from build123d import *

# Parameters (mm, degrees)
SKETCH1_W            = 202.5
SKETCH1_H            = 75
BOSS_EXTRUDE7_DEPTH  = 2.5
SKETCH9_W            = 10
SKETCH9_H            = 2.5
BOSS_EXTRUDE8_DEPTH  = 2.5
SKETCH10_W           = 10
SKETCH10_H           = 2.5
BOSS_EXTRUDE9_DEPTH  = 2.5
SKETCH11_R           = 1.5
CUT_EXTRUDE3_DEPTH   = 2.5
SKETCH12_W           = 2.5
SKETCH12_H           = 55
BOSS_EXTRUDE10_DEPTH = 2.5
SKETCH13_W           = 2.5
SKETCH13_H           = 55
BOSS_EXTRUDE11_DEPTH = 3


with BuildPart() as part:
    # Sketch1 → Boss-Extrude7 (new body)
    with BuildSketch(Plane.XY):
        with Locations((101.25, 37.5)):
            Rectangle(SKETCH1_W, SKETCH1_H)
    extrude(amount=BOSS_EXTRUDE7_DEPTH)

    # Sketch9 → Boss-Extrude8 (add)
    with BuildSketch(Plane(origin=(0, 75, 0), x_dir=(1, 0, 0), z_dir=(0, 1, 0))):
        with Locations((197.5, -1.25)):
            Rectangle(SKETCH9_W, SKETCH9_H)
    extrude(amount=BOSS_EXTRUDE8_DEPTH)

    # Sketch10 → Boss-Extrude9 (add)
    with BuildSketch(Plane.XZ):
        with Locations((197.5, 1.25)):
            Rectangle(SKETCH10_W, SKETCH10_H)
    extrude(amount=BOSS_EXTRUDE9_DEPTH)

    # Sketch11 → Cut-Extrude3 (cut)
    with BuildSketch(Plane.XY.offset(2.5)):
        with Locations((188.75, 37.5)):
            Circle(SKETCH11_R)
    extrude(amount=-CUT_EXTRUDE3_DEPTH, mode=Mode.SUBTRACT)

    # Sketch12 → Boss-Extrude10 (add)
    with BuildSketch(Plane(origin=(0, 0, 0), x_dir=(-1, 0, 0), z_dir=(0, 0, -1))):
        with Locations((-1.25, 37.5)):
            Rectangle(SKETCH12_W, SKETCH12_H)
    extrude(amount=BOSS_EXTRUDE10_DEPTH)

    # Sketch13 → Boss-Extrude11 (add)
    with BuildSketch(Plane.ZY):
        with Locations((-1.25, 37.5)):
            Rectangle(SKETCH13_W, SKETCH13_H)
    extrude(amount=BOSS_EXTRUDE11_DEPTH)


solid = part.part
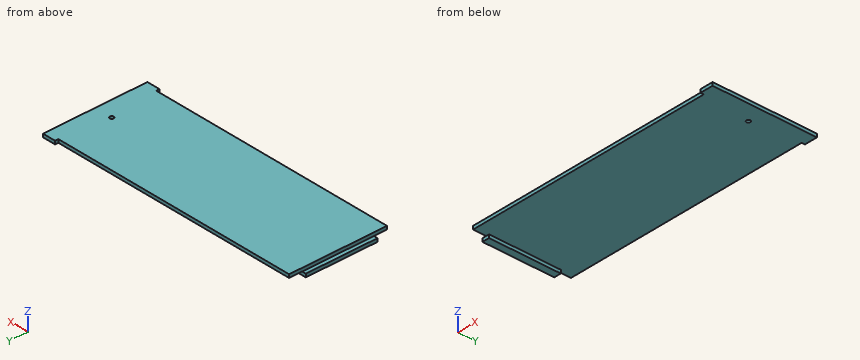
Source: CAD feature listing. Evaluate the final solid. Frame: model axes, mm. Give positions to 0.01 mm unless a question says otherwise; leave off trailing zeros. Write each loop counter-clockwise with the first axis right and the second up, starting at its lowest first coordinate (ties: lowest second). Pieces come first, ordered by that corner, then holes. Notation, with made-up numbers: M 67.5,64 L 79.5,64 A21 cw 79.5,83 Z; hole C 52.25,-1 d1. An arc over 180 degrees is marked long. Answer as a JSON object with one key per item and string values.
Q1. Cut plane A-A, the plane z = 0.9. Return the cut outline in (x, y).
Geometry check:
{"outline": "M 0,0 L 192.5,0 L 192.5,-2.5 L 202.5,-2.5 L 202.5,77.5 L 192.5,77.5 L 192.5,75 L 0,75 Z; hole C 188.75,37.5 d3"}
Q2. Cut plane D-D, the plane y = 5. Return the cut outline in (x, z), then the cut area to 3 significant figures.
Geometry check:
{"outline": "M 0,0 L 202.5,0 L 202.5,2.5 L 0,2.5 Z", "area": "506 mm^2"}
Q3. Contact query for flat-ended pins moving along their axis: P1, Ø1.5, axis at x = -2, y = 46.5, coming from the +Z side; P2, Ø1.2, axis at x = -1, z = -1, coming from the +Y side; P3, Ø1, axis at x = 156.5, y = 46.5, coming from the -Z side. Output: stop coordinate, or through.
Geometry check:
{"P1": "stops at z = 0", "P2": "stops at y = 65", "P3": "stops at z = 0"}
Q4. Cut plane B-B, the plane y = 21. Return the cut outline in (x, z).
Geometry check:
{"outline": "M -3,-2.5 L 2.5,-2.5 L 2.5,0 L 202.5,0 L 202.5,2.5 L 0,2.5 L 0,0 L -3,0 Z"}
Q5. Cut plane C-C, the plane x = 68. Return the cut outline in (y, z).
Geometry check:
{"outline": "M 0,0 L 75,0 L 75,2.5 L 0,2.5 Z"}
Q6. Ray query, line 1 along Y through (x, z) = (188.75, 0.6); line 2 along Z through (x, y) = (155, 60.5); line 3 along X through (y, z) = (32, 0.05). Return the intervals inside material, ascending.
Geometry check:
{"line 1": "y = 0 to 36, 39 to 75", "line 2": "z = 0 to 2.5", "line 3": "x = 0 to 202.5"}
